Geometry check sheet. Reference: the model listing, model coordinates, mm. Face numbers are marked on the shaded views. A direction names the side the tool comes from. Give positions to 0.01 mm unless a question says otherwise; leave off trailing zeros. Loops run counter-clockwise (first coordinate to the right, second up) from the corner with the lowest first, then second, coordinate; pieces in that order, holes last. Notation, with made-up numbers: (-14.75, -4.5) -> (13.25, -4.5) arc R15 cw to (13.25, -0.5) -> close; hole circle Ø9 at (89, 39). An arc over 180 degrees is marked (long way). Answer in a Markdown table with one row per item. Add a question column.
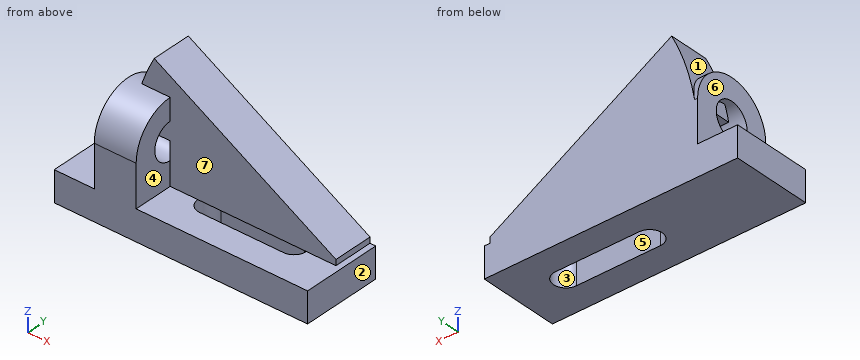
```python
from build123d import *

# Parameters (mm, degrees)
F0_W     = 42
F0_H     = 16
F1_DEPTH = 133
F2_START = 21
F0_R     = 9.5
F2_DEPTH = 22
F4_DEPTH = 25
F6_START = -21
F6_DEPTH = 21


with BuildPart() as f1:
    # F0 (on Right) → F1 (new body)
    with BuildSketch(Plane.YZ):
        with Locations((21, 8)):
            Rectangle(F0_W, F0_H)
    extrude(amount=F1_DEPTH)

    # F0 (on Right) → F2 (join)
    with BuildSketch(Plane.YZ.offset(F2_START)):
        with BuildLine():
            Line((0, 38), (0, 16))
            Line((0, 16), (42, 16))
            Line((42, 16), (42, 38))
            ThreePointArc((42, 38), (21, 59), (0, 38))
        make_face()
        with Locations((21, 38)):
            Circle(F0_R, mode=Mode.SUBTRACT)
    extrude(amount=F2_DEPTH)

    # F3 (on face) → F4 (cut)
    with BuildSketch(Plane.XY.offset(16)):
        with BuildLine():
            ThreePointArc((108, 14.5), (114.5, 21), (108, 27.5))
            Line((108, 27.5), (64, 27.5))
            ThreePointArc((64, 27.5), (57.5, 21), (64, 14.5))
            Line((64, 14.5), (108, 14.5))
        make_face()
    extrude(amount=-F4_DEPTH, mode=Mode.SUBTRACT)

    # F5 (on face) → F6 (join)
    with BuildSketch(Plane.XZ.offset(F6_START)):
        with BuildLine():
            Line((43, 16), (130, 16))
            Line((130, 16), (130, 19))
            Line((130, 19), (34.5883966818, 74.0859148596))
            ThreePointArc((34.5883966818, 74.0859148596), (27.1610557671, 56.5174050032), (22.5868188266, 38))
            Line((22.5868188266, 38), (43, 38))
            Line((43, 38), (43, 16))
        make_face()
    extrude(amount=-F6_DEPTH)


solid = f1.part
```
1. Material ranges on L1, parallel to Y at x = 91, z = 12; L2, parallel to X at y = 17, z = 51; L3, parallel to Y at x = 47, z = 42.5, recorded low to high. Write a range as from..to.
2. Sectioned sample at A-A (x = 73). Enter the section's corners in (y, z), plus the area to 3 significant figures.
3. Release check for a two-part mould opening along X. For the marked faces 1, 2 and 3 record: released by +X, released by -X, zero draft, split by the parting line, or undercut.
4. Sectioned sample at D-D (x = 40.5). Enter the section's corners in (y, z).
5. Access from +Z, -Z, +X, -X, +Y, -Y to the whole of each face (thin tool, end or side, straight path). Record for the marked faces 4, 5, 6 and 7.
6. Sectioned sample at C-C (y = 38.5). Enter the section's corners in (x, z), plus the area to 3 significant figures.
7. Gauge pin test, flat ends, axial feed: pin 1 Ø5 at (y, z) = (27, 35) entering from -X; pin 2 Ø8 at (y, z) = (20.5, 33.5) entering from +X; pin 3 Ø12.5 at (y, z) = (22.5, 47.5) entering from -X. Record the tip position at first contact, or that the pin passes through.
8. Sectioned sample at B-B (z = 45.5). Enter the section's corners in (x, y), plus the area to 3 significant figures.
Response:
| question | item | result |
|---|---|---|
| 1 | L1 | y = 0..14.5, 27.5..42 |
| 1 | L2 | x = 21..43 |
| 1 | L3 | y = 21..42 |
| 2 | outline | (0, 0) -> (14.5, 0) -> (14.5, 16) -> (0, 16) -> close; (21, 16) -> (27.5, 16) -> (27.5, 0) -> (42, 0) -> (42, 51.91) -> (21, 51.91) -> close |
| 2 | area | 1,220 mm2 |
| 3 | face 1 | released by -X |
| 3 | face 2 | released by +X |
| 3 | face 3 | undercut |
| 4 | outline | (0, 0) -> (42, 0) -> (42, 70.67) -> (21, 70.67) -> (21, 59) arc R21 ccw to (0, 38) -> close; hole (21, 38) -> (21, 47.5) arc R9.5 ccw (long way) to (30.5, 38) -> close |
| 5 | face 4 | +Z, +X, -Y |
| 5 | face 5 | +Z, -Z |
| 5 | face 6 | +Z, -X, +Y, -Y |
| 5 | face 7 | +X |
| 6 | outline | (0, 0) -> (133, 0) -> (133, 16) -> (130, 16) -> (130, 19) -> (34.59, 74.09) arc R121 ccw to (25.09, 49.61) -> (21, 49.61) -> (21, 16) -> (0, 16) -> close |
| 6 | area | 5,630 mm2 |
| 7 | pin 1 | stops at x = 43 |
| 7 | pin 2 | stops at x = 111.76 |
| 7 | pin 3 | stops at x = 21 |
| 8 | outline | (21, 1.38) -> (43, 1.38) -> (43, 15.17) -> (21, 15.17) -> close; (21, 26.83) -> (24.07, 26.83) -> (24.07, 21) -> (84.1, 21) -> (84.1, 42) -> (24.07, 42) -> (24.07, 40.62) -> (21, 40.62) -> close |
| 8 | area | 1,610 mm2 |
